from build123d import *

# Parameters (mm, degrees)
F0_R     = 31.75
F0_R_2   = 25.4
F1_DEPTH = 50.8
F0_R_3   = 3.3782
F2_DEPTH = 6.35


# Not quite as in the source:
# - a feature names something its author has since deleted; it is built from what else it names


with BuildPart() as f1:
    # F0 (on Right) → F1 (new body)
    with BuildSketch(Plane.YZ):
        Circle(F0_R)
        Circle(F0_R_2, mode=Mode.SUBTRACT)
    extrude(amount=F1_DEPTH)

    # F0 (on Right) → F2 (join)
    with BuildSketch(Plane.YZ):
        with BuildLine():
            Line((-48.0517219843, -7.1712400574), (-29.2791039707, -24.3791728874))
            ThreePointArc((-29.2791039707, -24.3791728874), (0, -38.1), (29.2791039707, -24.3791728874))
            Line((29.2791039707, -24.3791728874), (48.0517219843, -7.1712400574))
            ThreePointArc((48.0517219843, -7.1712400574), (51.2064, 0), (48.0517219843, 7.1712400574))
            Line((48.0517219843, 7.1712400574), (29.2791039707, 24.3791728874))
            ThreePointArc((29.2791039707, 24.3791728874), (0, 38.1), (-29.2791039707, 24.3791728874))
            Line((-29.2791039707, 24.3791728874), (-48.0517219843, 7.1712400574))
            ThreePointArc((-48.0517219843, 7.1712400574), (-51.2064, 0), (-48.0517219843, -7.1712400574))
        make_face()
        with Locations((-41.4782, 0)):
            Circle(F0_R_3, mode=Mode.SUBTRACT)
        Circle(F0_R, mode=Mode.SUBTRACT)
        with Locations((41.4782, 0)):
            Circle(F0_R_3, mode=Mode.SUBTRACT)
    extrude(amount=F2_DEPTH)


solid = f1.part
Build history of the part. All positions in model axes, mm. A direction names the side the tool comes from. Round coordinates to 2 decimals unless told otherwise and drop trailing zeros. Loops run counter-clockwise (first coordinate to the right, second up) from the corner with the lowest first, then second, coordinate; pieces in that order, holes last. Notation, with made-up numbers: (45.25, 76.5) -> (49.25, 76.5) arc R30 cw to (49.25, 105.5) -> close; hole circle Ø11 at (-9, 41). An arc over 180 degrees is marked (long way). Use CSV: the item, a comma, the result in double quotes. Start each with the question number.
Q1. Flat gauge pins, fed straight in: pin 1 Ø6 at (x, y) = (16.5, -20) entering from -Z; pin 2 Ø2 at (x, z) = (43, -19) entering from -Y; pin 3 Ø5 at (x, z) = (35, 2) entering from +Y; pin 4 Ø6 at (y, z) = (41.48, 0) entering from +X. Where does each tip first touch, or does it go through?
Q2. Mould opens along Z. For faces 3 (the face through (3.131, 0.467, 38.097)), 4 (the face through (28.264, -6.883, -30.995)), 5 (the face through (25.044, -5.506, -24.796)) say: +Z half, -Z half, draft (parallel to the pull), parting line (faces both ways), or undercut.
Q3. Saw through at B-B on y = 0. Give the cut face in (x, z).
Q4. Drill centre lines: L1, parallel to X at y = -34.5, z = -15; L2, parallel to Y at x = 23, z = -12; L3, parallel to Z at x = 34.5, y = -16.5. Where is each one in solid material? Low to high.
Q5. Saw through at C-C on x = 29. Give the cut face in (y, z), and give its area (3 significant figures).
Q6. Saw through at A-A on z = 0. Give the cut face in (x, y).
Q7. Which spindle directions (+Z, -Z, +X, -X, +Y, -Y) get a long thin tool onto all of the face, cutting with end or side? Do faces 1 (the face through (6.35, -8, -31)), 2 (the face through (3.131, -0.467, -38.097)). Say none if no direction does.
Q8. Saw through at D-D on z = 14. Give the cut face in (x, y).
Solutions:
1,pin 1,"stops at z = -26.82"
1,pin 2,"stops at y = -26.15"
1,pin 3,"stops at y = 31.75"
1,pin 4,"passes through"
2,face 3,"+Z half"
2,face 4,"parting line"
2,face 5,"undercut"
3,outline,"(0, -38.1) -> (6.35, -38.1) -> (6.35, -31.75) -> (50.8, -31.75) -> (50.8, -25.4) -> (0, -25.4) -> close; (0, 25.4) -> (50.8, 25.4) -> (50.8, 31.75) -> (6.35, 31.75) -> (6.35, 38.1) -> (0, 38.1) -> close"
4,L1,"x = 0 to 6.35"
4,L2,"y = -29.39 to -22.39, 22.39 to 29.39"
4,L3,"z = -27.13 to -19.31, 19.31 to 27.13"
5,outline,"circle Ø63.5 at (0, 0); hole circle Ø50.8 at (0, 0)"
5,area,"1,140 mm^2"
6,outline,"(0, -51.21) -> (6.35, -51.21) -> (6.35, -44.86) -> (0, -44.86) -> close; (0, -38.1) -> (6.35, -38.1) -> (6.35, -31.75) -> (50.8, -31.75) -> (50.8, -25.4) -> (0, -25.4) -> close; (0, 25.4) -> (50.8, 25.4) -> (50.8, 31.75) -> (6.35, 31.75) -> (6.35, 38.1) -> (0, 38.1) -> close; (0, 44.86) -> (6.35, 44.86) -> (6.35, 51.21) -> (0, 51.21) -> close"
7,face 1,"+X"
7,face 2,"-Z, +X, -X"
8,outline,"(0, -40.6) -> (6.35, -40.6) -> (6.35, -28.5) -> (50.8, -28.5) -> (50.8, -21.19) -> (0, -21.19) -> close; (0, 21.19) -> (50.8, 21.19) -> (50.8, 28.5) -> (6.35, 28.5) -> (6.35, 40.6) -> (0, 40.6) -> close"
